Autodesk Inventor part; units mm, degrees
ref_plane "YZ Plane" through (0, 0, 0) normal (1, 0, 0) x (0, 1, 0)
ref_plane "XZ Plane" through (0, 0, 0) normal (0, 1, 0) x (-1, 0, 0)
ref_plane "XY Plane" through (0, 0, 0) normal (0, 0, 1) x (1, 0, 0)
sketch "스케치1" plane through (0, 0, 0) normal (0, 0, 1) x (1, 0, 0)
  line L0 (-32.8, 35) -> (32.8, 35)
  line L1 (32.8, 35) -> (32.8, -35)
  line L2 (32.8, -35) -> (-32.8, -35)
  line L3 (-32.8, -35) -> (-32.8, 35)
  line L4 (-32.8, 35) -> (32.8, -35) construction
  line L5 (32.8, 35) -> (-32.8, -35) construction
  point P0 (0, 0)
  dimension "d0" = 65.6
  dimension "d1" = 70
extrude "돌출1" add sketch "스케치1" along normal blind 4
sketch "스케치2" plane through (32.8, -35, 0) normal (1, 0, 0) x (0, 0, -1)
  line L0 (0, 0) -> (0, 70)
  line L1 (0, 70) -> (-4, 70)
  line L2 (-4, 0) -> (-4, 70)
  line L3 (0, 0) -> (-4, 0)
  line L4 (0, 70) -> (-4, 70)
  line L5 (-2, 70) -> (-2, 0) construction
  line L6 (0, 0) -> (-4, 0)
  circle A0 centre (-2, 63) radius 1.25
  circle A1 centre (-2, 49) radius 1.25
  circle A2 centre (-2, 35) radius 1.25
  circle A3 centre (-2, 21) radius 1.25
  circle A4 centre (-2, 7) radius 1.25
  point P0 (0, 35)
  dimension "d4" = 2.5
  dimension "d5" = 2.5
  dimension "d6" = 2.5
  dimension "d8" = 2.5
  dimension "d9" = 2.5
  dimension "d10" = 14
  dimension "d11" = 7
  dimension "d12" = 14
  dimension "d13" = 7
  dimension "d14" = 14
extrude "돌출2" cut sketch "스케치2" against normal blind 6 contours A0 | A1 | A2 | A3 | A4
mirror "미러1" about plane through (0, 0, 0) normal (1, 0, 0) of "돌출2"
sketch "스케치3" plane through (0, 0, 0) normal (0, 0, -1) x (-1, 0, 0)
  line L0 (-18, 25) -> (18, 25)
  line L1 (18, 25) -> (18, -25)
  line L2 (18, -25) -> (-18, -25)
  line L3 (-18, -25) -> (-18, 25)
  line L4 (-18, 25) -> (18, -25) construction
  line L5 (18, 25) -> (-18, -25) construction
  point P0 (0, 0)
  dimension "d19" = 36
  dimension "d20" = 50
extrude "돌출3" cut sketch "스케치3" against normal blind 6
fillet "모깎기1" radius 6 4 edges at (18, 25, 2) (-18, 25, 2) (-18, -25, 2) (18, -25, 2)
properties part number "지지프레임2" material "알루미늄 6061"
Source: CAD feature listing. Evaluate the final solid. Frame: model axes, mm. A direction names the side the tool comes from. Give positions to 0.01 mm unless a question says otherwise; leave off trailing zeros. Write each loop counter-clockwise with the first axis right and the second up, starting at its lowest first coordinate (ties: lowest second). Pieces come first, ordered by that corner, then holes. Notation, with made-up numbers: M 45,79 L 95,79 A31 cw 95,107 Z; hole C 52.5,28 d1. An arc over 180 degrees is marked long. Return JSON: item names as keys, results as strings. Group by question number.
1) Pin query (flat end, axial travel): P1, Ø2, axis at y = 14, z = 2, coming from the -X side; P2, Ø1.2, axis at y = 0, z = 2.5, coming from the +X side. Return the tip coordinate at first contact, or that it passes through.
2) Cut plane B-B, the plane x = -7. Output: boundary loops of the cut face in (y, z), plus the area to 3 significant figures.
3) Cut plane C-C, the plane y = 28. Output: boundary loops of the cut face in (x, z).
4) Pull-direction query (Z, two-part tool) for faces 6 (the face through (18, 0, 2)), 7 (the face through (-22, 0, 4)), 8 (the face through (26.8, 0, 2)); classes: pulls with the +Z half, pulls with the -Z half, needs draft (parallel to the pull), parting line crosses it, or undercut.
5) Set-up query: faces 1 (the face through (-16.196, 23.289, 2.028)), 2 (the face through (32.8, 0.5, 0.6)), 3 (the face through (0, -35, 2)), 4 (the face through (-29.84, -28.38, 0.81)), 5 (the face through (26.8, 14, 2)). Return all of +Z, -Z, +X, -X, +Y, -Y with unobstructed straight access to the full face (end or side cutting, diameter ignored); none if empty.
6) Cut plane D-D, the plane y = 14. Output: boundary loops of the cut face in (x, z), plus the area to 3 significant figures.
7) Cut plane A-A, the plane y = 6.5. Output: boundary loops of the cut face in (x, z).
8) Material intervals for line 1 along Y through (x, z) = (29.25, 2); line 2 along Y through (x, z) = (11.5, 2.75); line 3 along X through (y, z) = (5, 2.15), sorted ascending. Write a range as [from, to].
Recorded:
{
 "1": {"P1": "stops at x = -26.8", "P2": "stops at x = 26.8"},
 "2": {"outline": "M -35,0 L -25,0 L -25,4 L -35,4 Z; M 25,0 L 35,0 L 35,4 L 25,4 Z", "area": "80.0 mm²"},
 "3": {"outline": "M -32.8,0 L 32.8,0 L 32.8,0.75 L 26.8,0.75 L 26.8,3.25 L 32.8,3.25 L 32.8,4 L -32.8,4 L -32.8,3.25 L -26.8,3.25 L -26.8,0.75 L -32.8,0.75 Z"},
 "4": {"face 6": "needs draft", "face 7": "pulls with the +Z half", "face 8": "undercut"},
 "5": {"face 1": "+Z, -Z", "face 2": "+Z, -Z, +X, +Y, -Y", "face 3": "+Z, -Z, +X, -X, -Y", "face 4": "-X", "face 5": "+X"},
 "6": {"outline": "M -32.8,0 L -18,0 L -18,4 L -32.8,4 L -32.8,3.25 L -26.8,3.25 L -26.8,0.75 L -32.8,0.75 Z; M 18,0 L 32.8,0 L 32.8,0.75 L 26.8,0.75 L 26.8,3.25 L 32.8,3.25 L 32.8,4 L 18,4 Z", "area": "88.4 mm²"},
 "7": {"outline": "M -32.8,0 L -18,0 L -18,4 L -32.8,4 Z; M 18,0 L 32.8,0 L 32.8,4 L 18,4 Z"},
 "8": {"line 1": "y = [-35, -29.25], [-26.75, -15.25], [-12.75, -1.25], [1.25, 12.75], [15.25, 26.75], [29.25, 35]", "line 2": "y = [-35, -25], [25, 35]", "line 3": "x = [-32.8, -18], [18, 32.8]"}
}
